Answer from the drawing. Dimensions are ordinates in mm from the lowest x, y and z of the part. A direction names the side the tool comes from. Give positions to 0.01 mm unless a question says otherwise; leave off trailing zeros. Loops run counter-clockwise (first coordinate to the right, second up) from the corner with the lowest first, then second, coordinate; pieces in that order, holes last. Notation, with made-up numbers: (6.5, 57.5) -> (20.5, 57.5) arc R7 cw to (20.5, 64.5) -> close; hole circle Ø5 at (-12, -11). An arc over 180 degrees is marked (long way). Answer as CSV lines item,"result". Start each with the question number.
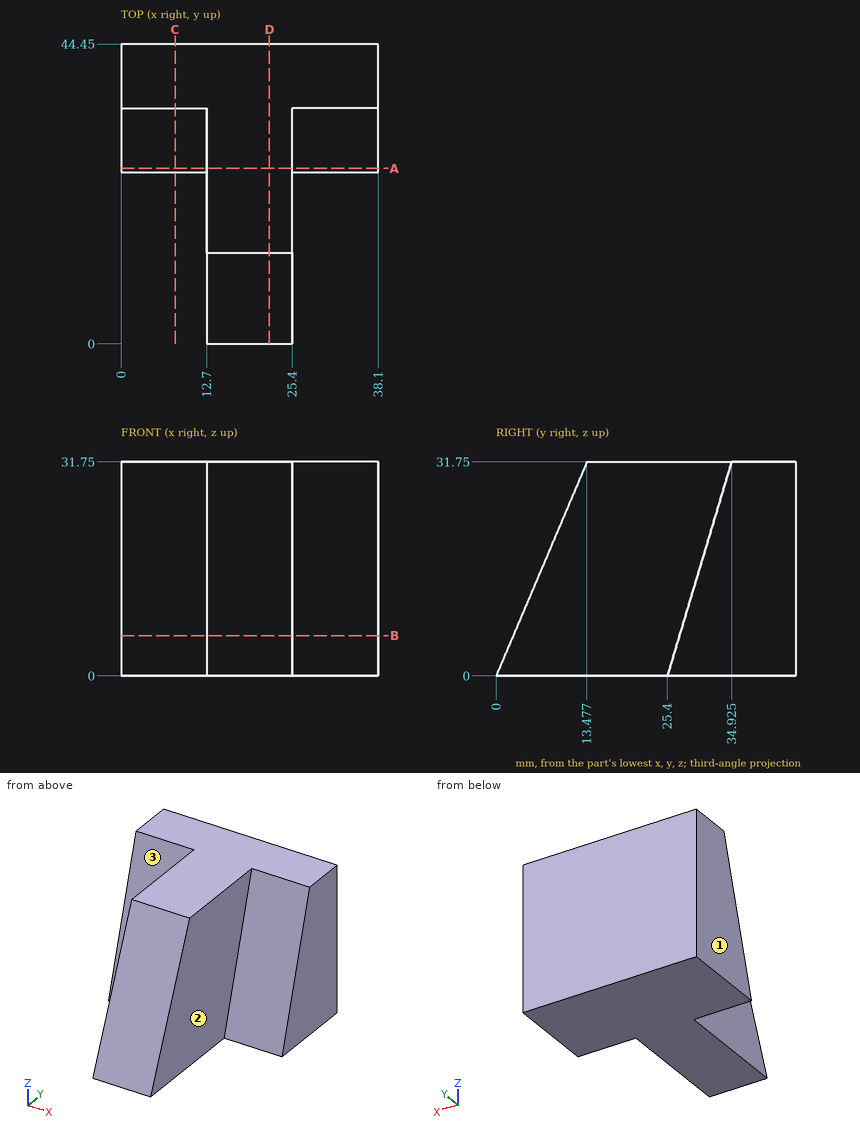
(1) A tool of negligible diameter and unlimited length cuts with its end or side. For the marked faces 1, 2 and 3, from which of +Z, -Z, +X, -X, +Y, -Y can it reach the whole face along a straight path? Write none if from no direction.
(2) Find section D-D on x = 22. Write down the section's boundary in (y, z), then the cut area to 3 significant figures.
(3) Find section C-C on x = 8. Write down the section's boundary in (y, z) (3 decimals).
(4) Find the intervals of material crossed by line 1 along X through (y, z) = (22.5, 20); line 2 along Y through (x, z) = (5, 10); line 3 along Y through (x, z) = (26, 24), in increasing order. Write a range as from..to.
(5) Find section A-A on y = 26. Write down the section's boundary in (x, z).
(6) Each of these flat-tipped pins is pushed along its axis until it touches: P1, Ø5, axis at x = 28.5, y = 13.5, coming from the +Z side; P2, Ø4, axis at x = 13, z = 13, coming from the -Y side. Where does it stop, or does it pass through?
(7) Find section B-B on z = 6. Write down the section's boundary in (x, y), then the cut area to 3 significant figures.
Answer block:
1,face 1,"+Z, -Z, -X, +Y, -Y"
1,face 2,"+Z, +X, -Y"
1,face 3,"+Z, -X, -Y"
2,outline,"(0, 0) -> (44.45, 0) -> (44.45, 31.75) -> (13.48, 31.75) -> close"
2,area,"1,200 mm2"
3,outline,"(25.4, 0) -> (44.45, 0) -> (44.45, 31.75) -> (34.925, 31.75) -> close"
4,line 1,"x = 12.7..25.4"
4,line 2,"y = 28.4..44.45"
4,line 3,"y = 32.6..44.45"
5,outline,"(0, 0) -> (38.1, 0) -> (38.1, 2) -> (25.4, 2) -> (25.4, 31.75) -> (12.7, 31.75) -> (12.7, 2) -> (0, 2) -> close"
6,P1,"passes through"
6,P2,"stops at y = 4.67"
7,outline,"(0, 27.2) -> (12.7, 27.2) -> (12.7, 2.55) -> (25.4, 2.55) -> (25.4, 27.2) -> (38.1, 27.2) -> (38.1, 44.45) -> (0, 44.45) -> close"
7,area,"970 mm2"
